```python
from build123d import *
from build123d.topology import SkipClean

# Parameters (mm, degrees)
CROQUIS1_R                  = 6
CROQUIS1_R_2                = 5
SALIENTE_EXTRUIR1_DEPTH     = 10
SALIENTE_EXTRUIR2_START     = -7
CROQUIS2_R                  = 5
CROQUIS2_R_2                = 2.5
SALIENTE_EXTRUIR2_DEPTH     = 7
CORTAR_EXTRUIR2_START       = -3.5
CROQUIS3_R                  = 5
CORTAR_EXTRUIR2_DEPTH       = 3.5
CROQUIS4_R                  = 6
CORTAR_EXTRUIR3_DEPTH       = 0.8
SALIENTE_EXTRUIR3_START     = -10
CROQUIS5_R                  = 7.5
CROQUIS5_R_2                = 5
SALIENTE_EXTRUIR3_DEPTH     = 10
SALIENTE_EXTRUIR4_START     = -8
SALIENTE_EXTRUIR4_DEPTH     = 8
CROQUIS7_W                  = 75
CROQUIS7_H                  = 7.168726593
SALIENTE_EXTRUIR5_DEPTH     = 90
SALIENTE_EXTRUIR6_DEPTH     = 7.168727
SALIENTE_EXTRUIR9_DEPTH     = 41
SALIENTE_EXTRUIR10_DEPTH    = 49
CORTAR_EXTRUIR4_START       = -41
CORTAR_EXTRUIR4_DEPTH       = 41
CORTAR_EXTRUIR5_DEPTH       = 143.675260973
CORTAR_EXTRUIR7_DEPTH       = 145.942427149
CORTAR_EXTRUIR8_DEPTH       = 145.942427149
CORTAR_EXTRUIR9_DEPTH       = 144.33727388
CROQUIS17_W                 = 30
CROQUIS17_H                 = 20.5
SALIENTE_EXTRUIR12_DEPTH    = 7.168727
CORTAR_EXTRUIR10_DEPTH      = 170.800324178
SALIENTE_EXTRUIR13_DEPTH    = 7.168723
SALIENTE_EXTRUIR14_DEPTH    = 7.168723
CORTAR_EXTRUIR12_DEPTH      = 171.613176039
CORTAR_EXTRUIR12_DEPTH_BACK = 171.613176039
SALIENTE_EXTRUIR15_DEPTH    = 7.168727
SALIENTE_EXTRUIR16_DEPTH    = 7.168727
SALIENTE_EXTRUIR17_DEPTH    = 2.399783
CORTAR_EXTRUIR13_DEPTH      = 165.428416042
CORTAR_EXTRUIR14_DEPTH      = 165.428416042
CORTAR_EXTRUIR15_DEPTH      = 150.41186397
CORTAR_EXTRUIR16_DEPTH      = 159.45665044


with BuildPart() as part:
    # Croquis1 → Saliente-Extruir1 (new body)
    with BuildSketch(Plane.XY):
        with Locations((10, 0)):
            Circle(CROQUIS1_R)
        with Locations((10, 0)):
            Circle(CROQUIS1_R_2, mode=Mode.SUBTRACT)
    extrude(amount=SALIENTE_EXTRUIR1_DEPTH)

    # Croquis2 → Saliente-Extruir2 (add)
    with BuildSketch(Plane.XY.offset(10).offset(SALIENTE_EXTRUIR2_START)):
        with Locations((10, 0)):
            Circle(CROQUIS2_R)
        with Locations((10, 0)):
            Circle(CROQUIS2_R_2, mode=Mode.SUBTRACT)
    extrude(amount=SALIENTE_EXTRUIR2_DEPTH)

    # Croquis3 → Cortar-Extruir2 (cut)
    with BuildSketch(Plane.XY.offset(10).offset(CORTAR_EXTRUIR2_START)):
        with Locations((10, 0)):
            Circle(CROQUIS3_R)
    extrude(amount=CORTAR_EXTRUIR2_DEPTH, mode=Mode.SUBTRACT)

    # Croquis4 → Cortar-Extruir3 (cut)
    with BuildSketch(Plane(origin=(0, 0, 0), x_dir=(-1, 0, 0), z_dir=(0, 0, -1))):
        with Locations((-10, 0)):
            Circle(CROQUIS4_R)
    extrude(amount=-CORTAR_EXTRUIR3_DEPTH, mode=Mode.SUBTRACT)

    # Croquis5 → Saliente-Extruir3 (add)
    with BuildSketch(Plane.XY.offset(10).offset(SALIENTE_EXTRUIR3_START)):
        with Locations((10, 0)):
            Circle(CROQUIS5_R)
        with Locations((10, 0)):
            Circle(CROQUIS5_R_2, mode=Mode.SUBTRACT)
    extrude(amount=SALIENTE_EXTRUIR3_DEPTH)

    # Croquis6 → Saliente-Extruir4 (add)
    with BuildSketch(Plane.XY.offset(10).offset(SALIENTE_EXTRUIR4_START)):
        with BuildLine():
            Line((-41.267602672, -17.548326339), (6.612435502, 6.691368079))
            ThreePointArc((6.612435502, 6.691368079), (3.071368624, -2.871248378), (12.338451231, -7.126124181))
            Line((12.338451231, -7.126124181), (-41.267602672, -24.717052932))
            Line((-41.267602672, -24.717052932), (-41.267602672, -17.548326339))
        make_face()
    extrude(amount=SALIENTE_EXTRUIR4_DEPTH)

    # Croquis7 → Saliente-Extruir5 (add)
    with BuildSketch(Plane.XY.offset(10)):
        with Locations((-78.767602672, -21.132689636)):
            Rectangle(CROQUIS7_W, CROQUIS7_H)
    extrude(amount=-SALIENTE_EXTRUIR5_DEPTH)

    # Croquis8 → Saliente-Extruir6 (add)
    with SkipClean():  # the faces are left unmerged after this step: merging them gives an invalid solid
        with BuildSketch(Plane.XZ.offset(24.717052932)):
            Polygon((-27.979148649, 2), (-41.267602672, -39), (-41.267602672, 2), align=None)
        extrude(amount=-SALIENTE_EXTRUIR6_DEPTH)

    # Croquis10 → Saliente-Extruir9 (add)
    with BuildSketch(Plane(origin=(0, 0, 2), x_dir=(-1, 0, 0), z_dir=(0, 0, -1))):
        Polygon((41.267602672, -17.548326339), (27.979148649, -17.548326339), (27.979148649, -10.820928511), align=None)
    extrude(amount=SALIENTE_EXTRUIR9_DEPTH)

    # Croquis11 → Saliente-Extruir10 (add)
    with BuildSketch(Plane(origin=(0, 0, -39), x_dir=(-1, 0, 0), z_dir=(0, 0, -1))):
        Polygon((41.267602672, -17.548326339), (41.267602672, -24.717052932), (27.979148649, -20.356421419), (27.979148649, -17.548326339), align=None)
    extrude(amount=-SALIENTE_EXTRUIR10_DEPTH)

    # Croquis12 → Cortar-Extruir4 (cut)
    with BuildSketch(Plane.XY.offset(2).offset(CORTAR_EXTRUIR4_START)):
        Polygon((-41.267602672, -24.717052932), (-27.979148649, -20.356421419), (-27.979148649, -24.717052932), align=None)
    extrude(amount=CORTAR_EXTRUIR4_DEPTH, mode=Mode.SUBTRACT)

    # Croquis13 → Cortar-Extruir5 (cut, through all)
    with BuildSketch(Plane(origin=(-1.347459035, 2.6616008, 0), x_dir=(0.89218241056854, 0.45167526639402034, 0), z_dir=(-0.45167526639402034, 0.89218241056854, 0))):
        Polygon((-29.850050056, -2), (-37.29721213, 39), (-29.850050056, 39), align=None)
    extrude(amount=-CORTAR_EXTRUIR5_DEPTH, mode=Mode.SUBTRACT)

    # Croquis14 → Cortar-Extruir7 (cut, through all)
    with BuildSketch(Plane(origin=(3.310603082, -10.088629756, 0), x_dir=(0.9501498907741007, 0.31179349746581414, 0), z_dir=(0.3117934974658141, -0.9501498907741006, 0))):
        Polygon((-29.95828018, 2), (-32.931384863, 2), (-36.10801617, -39), align=None)
    extrude(amount=-CORTAR_EXTRUIR7_DEPTH, mode=Mode.SUBTRACT)


with BuildPart() as cortar_extruir7_piece_1:
    # of the separate pieces the step leaves, piece 1, a body of its own (cortar_extruir7_pieces)
    add(part.part.solids().sort_by_distance((12.338451231, -7.126124181, 10))[0])


with BuildPart() as cortar_extruir7_piece_2:
    # of the separate pieces the step leaves, piece 2, a body of its own (cortar_extruir7_pieces)
    add(part.part.solids().sort_by_distance((-27.979148649, -20.356421419, -21.711689973))[0])


with BuildPart() as cortar_extruir8_tool:
    # Croquis15 → Cortar-Extruir8 (new, through all)
    with BuildSketch(Plane(origin=(3.310603082, -10.088629756, 0), x_dir=(0.9501498907741007, 0.31179349746581414, 0), z_dir=(0.3117934974658141, -0.9501498907741006, 0))):
        Polygon((-26.166370626, 2), (-33.745414131, 2), (-39.42969676, -39), (-33.745414131, -39), align=None)
    extrude(amount=-CORTAR_EXTRUIR8_DEPTH)


with BuildPart() as cortar_extruir7_piece_1_1:
    add(cortar_extruir7_piece_1.part)

    # Cortar-Extruir8: cut by cortar_extruir8_tool
    add(cortar_extruir8_tool.part, mode=Mode.SUBTRACT)

    # Croquis16 → Cortar-Extruir9 (cut, through all)
    with BuildSketch(Plane(origin=(0, -17.548326339, 0), x_dir=(1, 0, 0), z_dir=(0, 1, 0))):
        Polygon((-41.267602672, -10), (-46.041400107, 28.151463514), (-116.267602672, 39), (-116.267602672, -10), align=None)
    extrude(amount=-CORTAR_EXTRUIR9_DEPTH, mode=Mode.SUBTRACT)

    # Croquis17 → Saliente-Extruir12 (add)
    with SkipClean():  # the faces are left unmerged after this step: merging them gives an invalid solid
        with BuildSketch(Plane.XZ.offset(24.717052932)):
            with Locations((-131.267602672, -49.25)):
                Rectangle(CROQUIS17_W, CROQUIS17_H)
        extrude(amount=-SALIENTE_EXTRUIR12_DEPTH)

    # Croquis18 → Cortar-Extruir10 (cut, through all)
    with SkipClean():  # the faces are left unmerged after this step: merging them gives an invalid solid
        with BuildSketch(Plane.XZ.offset(24.717052932)):
            Polygon((-146.267602672, -59.5), (-116.267602672, -59.5), (-146.267602672, -64.144245374), align=None)
            Polygon((-116.267602672, -39), (-146.267602672, -43.634396888), (-146.267602672, -39), align=None)
        extrude(amount=-CORTAR_EXTRUIR10_DEPTH, mode=Mode.SUBTRACT)

    # Croquis19 → Saliente-Extruir13 (add)
    with SkipClean():  # the faces are left unmerged after this step: merging them gives an invalid solid
        with BuildSketch(Plane.XZ.offset(24.717052932)):
            Polygon((-146.267602672, -59.5), (-116.267602672, -59.5), (-146.267602672, -64.134396888), align=None)
        extrude(amount=-SALIENTE_EXTRUIR13_DEPTH)

    # Croquis20 → Saliente-Extruir14 (add)
    with SkipClean():  # the faces are left unmerged after this step: merging them gives an invalid solid
        with BuildSketch(Plane.XZ.offset(24.717052932)):
            Polygon((-146.267602672, -64.134396888), (-116.267602672, -59.5), (-116.267602672, -66.5), (-146.267602672, -71.134396888), align=None)
        extrude(amount=-SALIENTE_EXTRUIR14_DEPTH)

    # Simetría5: Cortar-Extruir7 piece 1 across plane


with BuildPart() as cortar_extruir7_piece_2_1:
    add(cortar_extruir7_piece_2.part)

    # Cortar-Extruir8: cut by cortar_extruir8_tool
    add(cortar_extruir8_tool.part, mode=Mode.SUBTRACT)


with BuildPart() as cortar_extruir7_piece_1_2:
    with SkipClean():  # the faces are left unmerged after this step: merging them gives an invalid solid
        add(cortar_extruir7_piece_1_1.part)
        add(cortar_extruir7_piece_1_1.part.mirror(Plane(origin=(-41.267602672, -24.717052932, -80), x_dir=(0, 0, 1), z_dir=(0, 1, 0))))

    # Croquis22 → Cortar-Extruir12 (cut, two sides: drawn at the far end of the back side and taken through both)
    with SkipClean():  # the faces are left unmerged after this step: merging them gives an invalid solid
        with BuildSketch(Plane(origin=(3.174348647, 0, -20.548619752), x_dir=(0.988277380271317, 0, 0.15266898717179916), z_dir=(-0.15266898717179916, 0, 0.988277380271317)).offset(-CORTAR_EXTRUIR12_DEPTH_BACK)):
            Polygon((-151.214582366, -24.717052932), (-160.929410211, -24.717052932), (-160.929410211, 29.151790767), (25.906832494, 29.151790767), (25.906832494, -24.717052932), align=None)
        extrude(amount=CORTAR_EXTRUIR12_DEPTH + CORTAR_EXTRUIR12_DEPTH_BACK, mode=Mode.SUBTRACT)

    # Croquis25 → Saliente-Extruir15 (add)
    with SkipClean():  # the faces are left unmerged after this step: merging them gives an invalid solid
        with BuildSketch(Plane.XZ.offset(31.885779526)):
            Polygon((-43.654501389, -9.075731757), (-64.181393268, -30.953727775), (-46.041400107, -28.151463514), align=None)
        extrude(amount=-SALIENTE_EXTRUIR15_DEPTH)

    # Croquis26 → Saliente-Extruir16 (add)
    with SkipClean():  # the faces are left unmerged after this step: merging them gives an invalid solid
        with BuildSketch(Plane.XZ.offset(31.885779526)):
            Polygon((-34.153518988, -39), (-41.267602672, -46.58234103), (-41.267602672, -39), align=None)
        extrude(amount=-SALIENTE_EXTRUIR16_DEPTH)

    # Croquis27 → Saliente-Extruir17 (add)
    with SkipClean():  # the faces are left unmerged after this step: merging them gives an invalid solid
        with BuildSketch(Plane.XZ.offset(31.885779526)):
            Polygon((-41.267602672, -39), (-34.153518988, -39), (-41.267602672, -46.58234103), align=None)
        extrude(amount=SALIENTE_EXTRUIR17_DEPTH)

    # Croquis28 → Cortar-Extruir13 (cut, through all)
    with SkipClean():  # the faces are left unmerged after this step: merging them gives an invalid solid
        with BuildSketch(Plane.XY.offset(-39)):
            Polygon((-41.267602672, -31.885779526), (-41.267602672, -34.285562838), (-36.527373087, -34.285562838), align=None)
            Polygon((-41.267602672, -24.717052932), (-34.153518988, -24.717052932), (-34.153518988, -27.051553051), align=None)
        extrude(amount=-CORTAR_EXTRUIR13_DEPTH, mode=Mode.SUBTRACT)

    # Croquis29 → Cortar-Extruir14 (cut, through all)
    with SkipClean():  # the faces are left unmerged after this step: merging them gives an invalid solid
        with BuildSketch(Plane.XY.offset(-39)):
            Polygon((-34.153518988, -27.051553051), (-36.527373087, -34.285562838), (-34.153518988, -34.285562838), align=None)
        extrude(amount=-CORTAR_EXTRUIR14_DEPTH, mode=Mode.SUBTRACT)

    # Croquis30 → Cortar-Extruir15 (cut, through all)
    with SkipClean():  # the faces are left unmerged after this step: merging them gives an invalid solid
        with BuildSketch(Plane(origin=(-21.268253266, -42.010627722, 0), x_dir=(0.8921824105685466, -0.4516752663940073, 0), z_dir=(-0.4516752663940073, -0.8921824105685466, 0))):
            Polygon((-17.103139044, -39), (-17.103139044, -41.530103964), (-17.512588728, -41.919452496), align=None)
        extrude(amount=-CORTAR_EXTRUIR15_DEPTH, mode=Mode.SUBTRACT)

    # Croquis33 → Cortar-Extruir16 (cut, through all)
    with SkipClean():  # the faces are left unmerged after this step: merging them gives an invalid solid
        with BuildSketch(Plane(origin=(-11.334278343, -34.539730358, 0), x_dir=(0.9501498907741053, -0.31179349746580015, 0), z_dir=(0.31179349746580015, 0.9501498907741053, 0))):
            Polygon((-24.016463998, 39), (-24.421219928, 41.919452496), (-24.016463998, 40.933309055), align=None)
        extrude(amount=-CORTAR_EXTRUIR16_DEPTH, mode=Mode.SUBTRACT)


solid = cortar_extruir7_piece_1_2.part
```
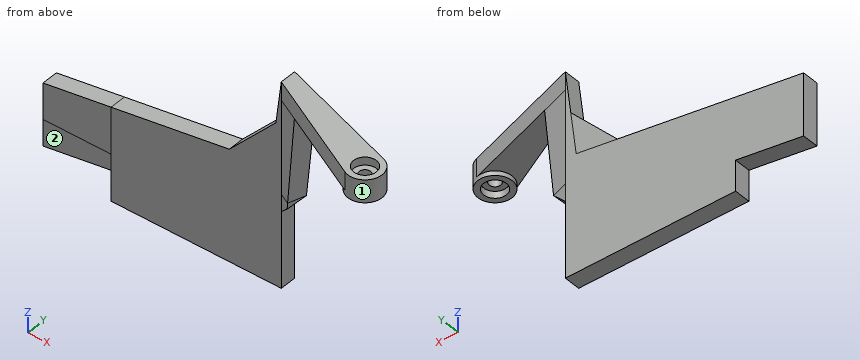
The model under review builds one solid part; all positions refer to its coordinate system, in mm. Face numbers are marked on the shaded views. A direction names the side the tool comes from. Give positions to 0.01 mm unless a question says otherwise; leave off trailing zeros. Write each loop counter-clockwise with the first axis right and the second up, starting at its lowest first coordinate (ties: lowest second). Pieces come first, ordered by that corner, then holes.
(1) Tool access review of the marked faces 1 and 2: name each direction out of +Z, -Z, +X, -X, +Y, -Y from which nothing blocks a thin tool from reaching the whole face with its end or side.
(2) Consider section A-A, the plane x = 10. Give the boundary of the cut face in (y, z).
(3) To check wall thickness, follow L1, parallel to Y at x = -116, z = -52; L2, parallel to Z at x = 2, y = -52; L3, parallel to Y at x = 10, z = 8.85. State the ranges of each line that lie inside material, in increasing order.
(4) For P1, Ø16.5, axis at x = -126, z = -50.5, coming from the -Y side; P2, Ø2, axis at y = -30, z = -68.5, coming from the +X side; P3, Ø5, axis at x = 12, y = -48, coming from the -Z side, all flat-tipped, find the tip position at first contact; note any pin that passes through.
(5) Consider section B-B, the plane z = -56.5. Give the boundary of the cut face in (x, y), and give its area (3 significant figures).
(6) Consider section D-D, the plane z = -14.5. Give the boundary of the cut face in (x, y).
Returned:
1. face 1: -Z
1. face 2: +Z, -Z, +X, -X, -Y
2. outline: (-56.93, 0) - (-54.43, 0) - (-54.43, 3) - (-51.93, 3) - (-51.93, 6.5) - (-54.43, 6.5) - (-54.43, 10) - (-56.93, 10) - close; (-46.93, 3) - (-44.43, 3) - (-44.43, 0) - (-41.93, 0) - (-41.93, 2) - (-41.54, 2) - (-41.54, 10) - (-44.43, 10) - (-44.43, 6.5) - (-46.93, 6.5) - close
3. L1: y = -31.89 to -24.72
3. L2: z = 2 to 10
3. L3: y = -56.93 to -54.43, -44.43 to -41.54
4. P1: stops at y = -31.89
4. P2: stops at x = -41.27
4. P3: stops at z = 3
5. outline: (-146.27, -31.89) - (-41.27, -31.89) - (-41.27, -24.72) - (-146.27, -24.72) - close
5. area: 753 mm2
6. outline: (-48.74, -31.89) - (-41.27, -31.89) - (-33.46, -35.84) - (-30.93, -28.11) - (-41.27, -24.72) - (-48.74, -24.72) - close
